from build123d import *

# Parameters (mm, degrees)
FILLET1_R                            = 1.016
BOSS_EXTRUDE1_START                  = -2.54
SKETCH2_R                            = 13.1445
SKETCH2_R_2                          = 12.954
BOSS_EXTRUDE1_DEPTH                  = 2.54
CUT_EXTRUDE1_START                   = -0.508
SKETCH3_R                            = 7.493
CUT_EXTRUDE1_DEPTH                   = 0.508
CUT_EXTRUDE2_START                   = -3.302
CUT_EXTRUDE2_DEPTH                   = 3.302
RIB1_REACH                           = 25.878
SKETCH7_WALL_W                       = 52.380916808
SKETCH7_WALL_H                       = 1.524
BOSS_EXTRUDE2_REACH                  = 32.187
SKETCH9_W                            = 1.524
SKETCH9_H                            = 6.096
BOSS_EXTRUDE2_DIRECTION_2_REACH      = 32.187
BOSS_EXTRUDE2_DIRECTION_2_END_RADIUS = 9.525


# Read off the part's stored shape, not the designer's step: Draft1
with BuildPart() as part:
    # Sketch1 → Base-Revolve (revolve)
    with BuildSketch(Plane.XY, mode=Mode.PRIVATE) as base_revolve_sk:
        Polygon((12.954, 3.819921875), (12.954, 14.986), (7.493, 14.986), (7.493, 5.842), (3.175, 5.842), (3.175, 11.684), (2.032, 11.684), (2.032, 3.302), (7.493, 3.302), (7.493, 0), (9.525, 0), (9.525, 12.963921875), (11.938, 12.963921875), (11.938, 3.819921875), align=None)
    revolve(base_revolve_sk.sketch.rotate(Axis((0, 0, 0), (0, 1, 0)), 90), axis=Axis((0, 0, 0), (0, 1, 0)))

    # Fillet1
    fillet1_edges = [part.edges().sort_by_distance(p)[0] for p in [
        (0, 14.986, 12.954),
    ]]
    fillet(fillet1_edges, radius=FILLET1_R)

    # Sketch2 → Boss-Extrude1 (add)
    with BuildSketch(Plane.XZ.offset(-3.819921875).offset(BOSS_EXTRUDE1_START)):
        with Locations(Location((0, 0, 0), (0, 0, 270))):
            Circle(SKETCH2_R)
        with Locations(Location((0, 0, 0), (0, 0, 270))):
            Circle(SKETCH2_R_2, mode=Mode.SUBTRACT)
    extrude(amount=BOSS_EXTRUDE1_DEPTH)

    # Sketch3 → Cut-Extrude1 (cut)
    with BuildSketch(Plane(origin=(0, 14.986, 0), x_dir=(-1, 0, 0), z_dir=(0, 1, 0)).offset(CUT_EXTRUDE1_START)):
        with BuildLine():
            Line((1.27, -10.720033815), (1.27, -9.017))
            Line((1.27, -9.017), (-1.27, -9.017))
            Line((-1.27, -9.017), (-1.27, -10.720033815))
            ThreePointArc((-1.27, -10.720033815), (0, 10.795), (1.27, -10.720033815))
        make_face()
        with Locations(Location((0, 0, 0), (0, 0, 270))):
            Circle(SKETCH3_R, mode=Mode.SUBTRACT)
    extrude(amount=CUT_EXTRUDE1_DEPTH, mode=Mode.SUBTRACT)

    # Draft1 outline → Draft1 (revolve, cut)
    with BuildSketch(Plane.XY):
        Polygon((12.257315516, 3.819921875), (11.938, 12.963921875), (11.938, 3.819921875), align=None)
    revolve(axis=Axis((0, 0, 0), (0, 1, 0)), mode=Mode.SUBTRACT)

    # Sketch4 → Cut-Revolve1 (revolve, cut)
    with BuildSketch(Plane.XY, mode=Mode.PRIVATE) as cut_revolve1_sk:
        Polygon((9.525, 3.819921875), (9.144, 1.905), (8.89, 0), (9.525, 0), align=None)
    revolve(cut_revolve1_sk.sketch.rotate(Axis((0, 0, 0), (0, 1, 0)), 90), axis=Axis((0, 0, 0), (0, 1, 0)), mode=Mode.SUBTRACT)

    # Sketch5 → Boss-Revolve1 (revolve)
    with BuildSketch(Plane.XY, mode=Mode.PRIVATE) as boss_revolve1_sk:
        Polygon((2.032, 3.302), (2.032, 3.048), (3.556, 3.048), (3.556, 2.286), (5.969, 2.286), (5.969, 3.302), align=None)
    revolve(boss_revolve1_sk.sketch.rotate(Axis((0, 0, 0), (0, 1, 0)), 90), axis=Axis((0, 0, 0), (0, 1, 0)))

    # Sketch6 → Cut-Extrude2 (cut)
    with BuildSketch(Plane.XZ.offset(CUT_EXTRUDE2_START)):
        with BuildLine():
            Line((-6.174789514, 7.252420248), (-4.732067149, 5.809697884))
            ThreePointArc((-4.732067149, 5.809697884), (-5.298351111, 5.298351111), (-5.809697884, 4.732067149))
            Line((-5.809697884, 4.732067149), (-7.252420248, 6.174789514))
            ThreePointArc((-7.252420248, 6.174789514), (-6.735192091, 6.735192091), (-6.174789514, 7.252420248))
        make_face()
    extrude(amount=CUT_EXTRUDE2_DEPTH, mode=Mode.SUBTRACT)

    # Sketch7 wall → Rib1 (add, up to next)
    with BuildSketch(Plane(origin=(0, 6.867921875, 10.837938506), x_dir=(0, 0, -1), z_dir=(0, 1, 0)), mode=Mode.PRIVATE) as rib1_sk1:
        with Locations((0, -0.762)):
            Rectangle(SKETCH7_WALL_W, SKETCH7_WALL_H)
    rib1_tool1 = extrude(rib1_sk1.sketch, amount=RIB1_REACH, mode=Mode.PRIVATE) - part.part
    add(rib1_tool1.solids().sort_by_distance((0, 6.867921875, 10.837938506))[0])

    # Boss-Extrude2: up to this cone (the profile starts inside it)
    boss_extrude2_end = Plane(origin=(0, 9.915922, 0), z_dir=(0, -1, 0)) * Cone(10.482382248, 13.606494754, 89.462877002, mode=Mode.PRIVATE)
    # Sketch9 → Boss-Extrude2 (add, up to the surface)
    with BuildSketch(Plane.XY.offset(9.525), mode=Mode.PRIVATE) as boss_extrude2_sk1:
        with Locations((6.096, 9.915921875)):
            Rectangle(SKETCH9_W, SKETCH9_H)
    boss_extrude2_tool1 = extrude(boss_extrude2_sk1.sketch, amount=BOSS_EXTRUDE2_REACH, mode=Mode.PRIVATE) & boss_extrude2_end
    add(boss_extrude2_tool1.solids().sort_by_distance((6.096, 9.915922, 9.525))[0])

    # Boss-Extrude2 direction 2: up to this cylinder (the profile starts outside it)
    boss_extrude2_direction_2_end = Plane(origin=(0, 9.915922, 0), z_dir=(0, -1, 0)) * Cylinder(BOSS_EXTRUDE2_DIRECTION_2_END_RADIUS, 84.424, mode=Mode.PRIVATE)
    # Sketch9 → Boss-Extrude2 direction 2 (add, up to the surface)
    with BuildSketch(Plane.XY.offset(9.525), mode=Mode.PRIVATE) as boss_extrude2_direction_2_sk1:
        with Locations((6.096, 9.915921875)):
            Rectangle(SKETCH9_W, SKETCH9_H)
    boss_extrude2_direction_2_tool1 = extrude(boss_extrude2_direction_2_sk1.sketch, amount=-BOSS_EXTRUDE2_DIRECTION_2_REACH, mode=Mode.PRIVATE) - boss_extrude2_direction_2_end
    add(boss_extrude2_direction_2_tool1.solids().sort_by_distance((6.096, 9.915922, 9.525))[0])


solid = part.part
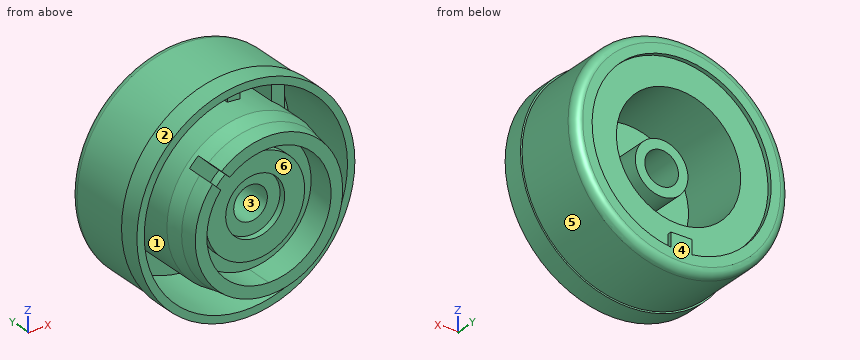
Work out the finished part from the listing and answer in its coordinate system (mm). Face numbers are marked on the shaded views. A direction names the side the tool comes from. Round coordinates to 2 decimals unless told otherwise and drop trailing zeros. Write each loop counter-clockwise with the first axis right and the second up, starting at its lowest first coordinate (ties: lowest second). Pieces come first, ordered by that corner, then holes.
1) A cutting plane is placed at A-A (y = 8.25). Give the vertices of the cut face in (x, z) (3 decimals).
2) A tool of negligible diameter and unlimited length cuts with its end or side. For the marked faces 5 and 6, from which of +Z, -Z, +X, -X, +Y, -Y can it reach the whole face along a straight path? Write none if from no direction.
3) Given pin 1 Ø1 at (x, z) = (-6.5, -1) entering from +Y; pin 2 Ø13.5 at (x, z) = (0, 0) entering from +Y; pin 3 Ø1.7 at (x, z) = (1, 10.5) entering from -Y, each flat-ended and moving along its own axis, determine where each tip first touches the part or whether it passes through.
4) The mould has two halves that part along X. Classify the marked faces 1, 2, 3 and 4: pulls with the +X half, pulls with the -X half, needs draft (parallel to the pull), parting line crosses it, or undercut.
5) Straight lines are drawn through the part: line 1 (X direction, y = 7.25, z = -0.75); line 2 (X direction, y = 5, z = 4); line 3 (Z direction, x = -0.5, y = 9.25). For each, find the intervals that lie inside material, in ascending order.
Completed:
1. outline: circle Ø25.908 at (0, 0); circle Ø6.35 at (0, 0); hole circle Ø14.986 at (0, 0); hole circle Ø4.064 at (0, 0); hole (0, 9.525) - (0, 12.103) arc R12.103 ccw (long way) to (6.858, 9.972) - (6.858, 6.61) arc R9.525 cw (long way) to start; hole (1.524, 9.402) arc R9.525 cw to (5.334, 7.891) - (5.334, 10.864) arc R12.103 ccw to (1.524, 12.006) - close
2. face 5: +Y
2. face 6: -Y
3. pin 1: stops at y = 5.84
3. pin 2: stops at y = 11.68
3. pin 3: stops at y = 6.87
4. face 1: undercut
4. face 2: parting line crosses it
4. face 3: undercut
4. face 4: needs draft
5. line 1: x = -12.93 to -12.11, -9.5 to -7.46, -3.09 to -1.89, 1.89 to 3.09, 7.46 to 9.5, 12.11 to 12.93
5. line 2: x = -12.52 to -11.54, -8.64 to 8.64, 11.54 to 12.52
5. line 3: z = -12.94 to -12.06, -9.51 to -7.48, -3.14 to -1.97, 1.97 to 3.14, 7.48 to 9.51, 12.06 to 12.94
